```python
from build123d import *

# Parameters (mm, degrees)
SKETCH1_W                  = 96
SKETCH1_H                  = 96
BOSS_EXTRUDE1_DEPTH        = 1.8
F_3_2_3_2_DIAMETER_HOLE1_D = 3.2


with BuildPart() as part:
    # Sketch1 → Boss-Extrude1 (new body)
    with BuildSketch(Plane.XY):
        Rectangle(SKETCH1_W, SKETCH1_H)
    extrude(amount=BOSS_EXTRUDE1_DEPTH)

    # Ø3.2 (3.2) Diameter Hole1 (through all)
    with Locations(Plane.XY.offset(1.8)):
        with Locations((39, -39)):
            Hole(F_3_2_3_2_DIAMETER_HOLE1_D / 2)


solid = part.part
```
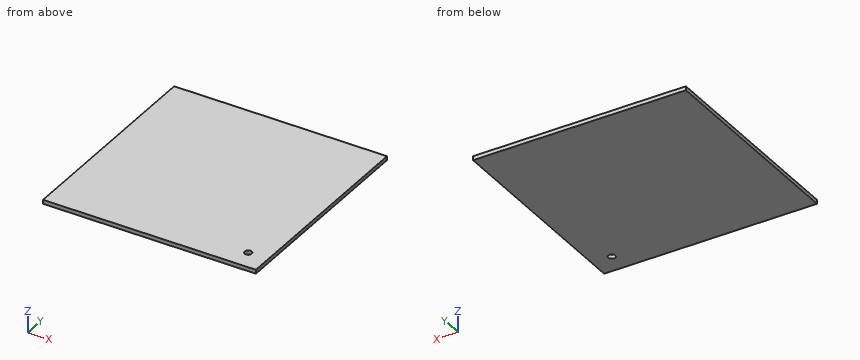
The model under review builds one solid part; all positions refer to its coordinate system, in mm. Round coordinates to 2 decimals unless told otherwise and drop trailing zeros. Write each loop counter-clockwise with the first axis right and the second up, starting at its lowest first coordinate (ties: lowest second). Pieces come first, ordered by that corner, then holes.
(1) Wall thickness on L1, parallel to Y at x = 39, z = 0.5: over which ranges is the line inside the solid? List them lowest first.
(2) We need section A-A on x = 39. Give the boundary of the cut face in (y, z), and give its area (3 significant figures).
(3) We need section B-B on y = -39. Give the boundary of the cut face in (x, z), and give its area (3 significant figures).
(4) Insertion check: pin 1 (3.5 mm diameter, centred on x = 39, y = -39, fed in from +Z). The pin has a flat end and moves straight along its axis. Give the tip position at first contact, or say it passes through.
Findings below:
1. L1: y = -48 to -40.6, -37.4 to 48
2. outline: (-48, 0) - (-40.6, 0) - (-40.6, 1.8) - (-48, 1.8) - close; (-37.4, 0) - (48, 0) - (48, 1.8) - (-37.4, 1.8) - close
2. area: 167 mm2
3. outline: (-48, 0) - (37.4, 0) - (37.4, 1.8) - (-48, 1.8) - close; (40.6, 0) - (48, 0) - (48, 1.8) - (40.6, 1.8) - close
3. area: 167 mm2
4. pin 1: stops at z = 1.8
